Input: part model. Units: mm. Frame: model coordinates. A direction names the side the tool comes from. Coordinates: 2 decimals unless noted, no trailing zeros. Loops run counter-clockwise (first coordinate to the right, second up) from the corner with the lowest first, then second, coordinate; pieces in that order, holes last.
```python
from build123d import *

# Parameters (mm, degrees)
ESQUISSE2_R             = 21.716757685
BOSS_EXTRU_1_DEPTH      = 1
ENL_V_MAT_EXTRU_2_DEPTH = 293.837814183
CONG_2_R                = 10


with BuildPart() as part:
    # Esquisse2 → Boss.-Extru.1 (new body)
    with BuildSketch(Plane.XY):
        with Locations((-43.22899501, 36.585487108)):
            Circle(ESQUISSE2_R)
        with BuildLine():
            ThreePointArc((-207.546192285, -7.001881243), (-132.259115873, 40.696309579), (-43.22899501, 36.585487108))
            ThreePointArc((-43.22899501, 36.585487108), (-84.183978752, -42.572270496), (-163.135361924, -83.923695834))
            ThreePointArc((-163.135361924, -83.923695834), (-190.453313653, -48.414512892), (-207.546192285, -7.001881243))
        make_face()
        with BuildLine():
            ThreePointArc((76.677371904, -83.923695834), (-2.274011269, -42.572270496), (-43.22899501, 36.585487108))
            ThreePointArc((-43.22899501, 36.585487108), (45.801125853, 40.696309579), (121.088202265, -7.001881243))
            ThreePointArc((121.088202265, -7.001881243), (103.995323633, -48.414512892), (76.677371904, -83.923695834))
        make_face()
        with BuildLine():
            Line((-43.22899501, 206.585487108), (-43.22899501, 58.302244794))
            ThreePointArc((-43.22899501, 58.302244794), (-34.753748483, 56.580180421), (-27.622617897, 51.687094896))
            ThreePointArc((-27.622617897, 51.687094896), (7.298277527, 122.217794206), (1.181835351, 200.682038403))
            ThreePointArc((1.181835351, 200.682038403), (-20.82825529, 205.103162324), (-43.22899501, 206.585487108))
        make_face()
        with BuildLine():
            ThreePointArc((-58.835372123, 51.687094896), (-51.704241537, 56.580180421), (-43.22899501, 58.302244794))
            Line((-43.22899501, 58.302244794), (-43.22899501, 206.585487108))
            ThreePointArc((-43.22899501, 206.585487108), (-65.62973473, 205.103162324), (-87.639825371, 200.682038403))
            ThreePointArc((-87.639825371, 200.682038403), (-93.756267547, 122.217794206), (-58.835372123, 51.687094896))
        make_face()
        with BuildLine():
            ThreePointArc((-48.504182436, 15.519164174), (-45.480177087, 25.955564863), (-43.22899501, 36.585487108))
            ThreePointArc((-43.22899501, 36.585487108), (-53.560368754, 39.950867364), (-64.110559549, 42.550202255))
            ThreePointArc((-64.110559549, 42.550202255), (-62.036258854, 25.727108266), (-48.504182436, 15.519164174))
        make_face()
        with BuildLine():
            ThreePointArc((-22.347430471, 42.550202255), (-32.897621267, 39.950867364), (-43.22899501, 36.585487108))
            ThreePointArc((-43.22899501, 36.585487108), (-40.977812933, 25.955564863), (-37.953807584, 15.519164174))
            ThreePointArc((-37.953807584, 15.519164174), (-26.109159563, 23.224020174), (-21.512237325, 36.585487108))
            ThreePointArc((-21.512237325, 36.585487108), (-21.722049137, 39.596939182), (-22.347430471, 42.550202255))
        make_face()
        with BuildLine():
            ThreePointArc((-37.953807584, 15.519164174), (-40.977812933, 25.955564863), (-43.22899501, 36.585487108))
            ThreePointArc((-43.22899501, 36.585487108), (-45.480177087, 25.955564863), (-48.504182436, 15.519164174))
            ThreePointArc((-48.504182436, 15.519164174), (-43.22899501, 14.868729423), (-37.953807584, 15.519164174))
        make_face()
        with BuildLine():
            ThreePointArc((-64.110559549, 42.550202255), (-53.560368754, 39.950867364), (-43.22899501, 36.585487108))
            ThreePointArc((-43.22899501, 36.585487108), (-51.309186676, 43.850029099), (-58.835372123, 51.687094896))
            ThreePointArc((-58.835372123, 51.687094896), (-62.036258854, 47.443865951), (-64.110559549, 42.550202255))
        make_face()
        with BuildLine():
            ThreePointArc((-58.835372123, 51.687094896), (-51.309186676, 43.850029099), (-43.22899501, 36.585487108))
            Line((-43.22899501, 36.585487108), (-43.22899501, 58.302244794))
            ThreePointArc((-43.22899501, 58.302244794), (-51.704241537, 56.580180421), (-58.835372123, 51.687094896))
        make_face()
        with BuildLine():
            Line((-43.22899501, 58.302244794), (-43.22899501, 36.585487108))
            ThreePointArc((-43.22899501, 36.585487108), (-35.148803344, 43.850029099), (-27.622617897, 51.687094896))
            ThreePointArc((-27.622617897, 51.687094896), (-34.753748483, 56.580180421), (-43.22899501, 58.302244794))
        make_face()
        with BuildLine():
            ThreePointArc((-27.622617897, 51.687094896), (-35.148803344, 43.850029099), (-43.22899501, 36.585487108))
            ThreePointArc((-43.22899501, 36.585487108), (-32.897621267, 39.950867364), (-22.347430471, 42.550202255))
            ThreePointArc((-22.347430471, 42.550202255), (-24.421731167, 47.443865951), (-27.622617897, 51.687094896))
        make_face()
    extrude(amount=BOSS_EXTRU_1_DEPTH)

    # Esquisse4 → Enlèv. mat.-Extru.2 (cut, through all)
    with BuildSketch(Plane(origin=(0, 0, 0), x_dir=(-1, 0, 0), z_dir=(0, 0, -1))):
        with BuildLine():
            Line((46.937094254, 35.085487108), (39.520895767, 35.085487108))
            ThreePointArc((39.520895767, 35.085487108), (43.22899501, 40.585487108), (46.937094254, 35.085487108))
        make_face()
    extrude(amount=-ENL_V_MAT_EXTRU_2_DEPTH, mode=Mode.SUBTRACT)

    # Congé2
    cong_2_edges = [part.edges().sort_by_distance(p)[0] for p in [
        (-87.639825371, 200.682038403, 0.5),
        (1.181835351, 200.682038403, 0.5),
        (121.088202265, -7.001881243, 0.5),
        (76.677371904, -83.923695834, 0.5),
        (-163.135361924, -83.923695834, 0.5),
        (-207.546192285, -7.001881243, 0.5),
    ]]
    fillet(cong_2_edges, radius=CONG_2_R)


solid = part.part
```
Item 1: Reachability of faces 5 (the face through (4.36, -48.84, 0.49)), 6 (the face through (52.5, 38.75, 0.49)), 7 (the face through (-46, 32, 1)) from +Z, -Z, +X, -X, +Y, -Y: full face, straight path, thin tool, end or side. Return the list, or none.
Result:
face 5: +Z, -Z, -Y
face 6: +Z, -Z
face 7: +Z, +X, -X, +Y, -Y
Item 2: Section query D-D (x = 56.5). Output: boundary loops of the cut face in (y, z), then the cut area to 3 significant figures.
Result:
outline: (-78.83, 0) - (37.42, 0) - (37.42, 1) - (-78.83, 1) - close
area: 116 mm2
Item 3: Section query B-B (x = -72). Output: boundary loops of the cut face in (y, z), then the cut area to 3 significant figures.
Result:
outline: (-28.7, 0) - (43.97, 0) - (43.97, 1) - (-28.7, 1) - close; (68.81, 0) - (204.13, 0) - (204.13, 1) - (68.81, 1) - close
area: 208 mm2
Item 4: Line query: L1, parallel to Y at x = -80.5, z = 0.5; L2, parallel to X at y = 9, z = 0.15; L3, parallel to Y at x = -41, z = 0.7. Output: solid intervals per line, ascending.
Result:
L1: y = -38.73 to 45.01, 83.47 to 202.45
L2: x = -191.83 to -50.83, -35.63 to 105.37
L3: y = 14.98 to 35.09, 39.91 to 206.57
Item 5: Section query A-A (y = -45). Output: boundary loops of the cut face in (x, z).
Result:
outline: (-192.37, 0) - (-86.66, 0) - (-86.66, 1) - (-192.37, 1) - close; (0.2, 0) - (105.91, 0) - (105.91, 1) - (0.2, 1) - close
Item 6: Section query C-C (y = 102). Output: boundary loops of the cut face in (x, z).
Result:
outline: (-88.34, 0) - (1.88, 0) - (1.88, 1) - (-88.34, 1) - close
Item 7: Mould query, pull axis X, two halves, no side actions, for faces 1 (the face through (6.51, 118.41, 0.49)), 2 (the face through (-141.009, 38.084, 0.493)), 3 (the face through (-89.22, -47.4, 0.49)), 4 (the face through (-93.417, 120.516, 0.493)). Classes: +X half, -X half, draft (parallel to the pull), parting line (faces both ways), or undercut.
Result:
face 1: +X half
face 2: undercut
face 3: undercut
face 4: -X half
